Input: part model. Units: mm. Frame: model coordinates. A direction names the side the tool comes from. Coordinates: 2 decimals unless noted, no trailing zeros. Loops run counter-clockwise (first coordinate to the right, second up) from the corner with the lowest first, then second, coordinate; pieces in that order, holes last.
Item 1: Reachability of faces 4 (the flat face through (1, 0, 8)), 5 (the flat face through (0, 3, -5.25)) from +Z, -Z, +X, -X, +Y, -Y: full face, straight path, thin tool, end or side. Return the list, or none.
Item 2: Section B-B on x = 29.75. Return loops of the section in (y, z), and give its area (3 significant figures).
Item 3: Section D-D on x = -16.5. Return loops of the section in (y, z).
Item 4: Section C-C on y = 2.2. Return loops of the section in (x, z), and give its area (3 significant figures).
Item 5: Section A-A on z = 0. Return loops of the section in (x, y), and give its area (3 significant figures).
Item 6: Contact query for flat-ended pins moving along their axis: P1, Ø1, axis at x = -44, y = 3.5, coming from the -Z side; P2, Ø1.6, axis at y = 2, z = 2, coming from the -X side; P3, Ø1.5, axis at x = 30, y = 4.5, coming from the -Z side. Output: stop coordinate, or through.
Item 7: Ray query, line 1 along X through (y, z) = (2.4, 0); line 2 along Z through (x, y) = (-3, 0.9); line 3 along Z through (x, y) = (-29.75, 1). Return the intervals inside material, ascending.
Item 8: Pull-direction query (X, two-part tool) for faces 1 (the cylindrical face through (55.322, 4.145, -0.487)), 2 (the flat face through (1, 5.5, 7)), 3 (the cylindrical face through (-27.554, 1.972, -0.488)); classes: released by +X, released by -X, zero draft, split by the parting line, or undercut.
Autodesk Inventor part; units mm, degrees
ref_plane "YZ Plane" through (0, 0, 0) normal (1, 0, 0) x (0, 1, 0)
ref_plane "XZ Plane" through (0, 0, 0) normal (0, 1, 0) x (-1, 0, 0)
ref_plane "XY Plane" through (0, 0, 0) normal (0, 0, 1) x (1, 0, 0)
sketch "Sketch1" plane through (0, 0, 0) normal (0, 1, 0) x (-1, 0, 0)
  line L0 (-56.75, -34.75) -> (56.75, -34.75)
  line L1 (56.75, -34.75) -> (56.75, 34.75)
  line L2 (56.75, 34.75) -> (-56.75, 34.75)
  line L3 (-56.75, 34.75) -> (-56.75, -34.75)
  line L4 (-56.75, -34.75) -> (56.75, 34.75) construction
  line L5 (56.75, -34.75) -> (-56.75, 34.75) construction
  point P0 (0, 0)
  dimension "d0" = 113.5
  dimension "d1" = 69.5
extrude "Extrusion1" add sketch "Sketch1" along normal blind 5.5
sketch "Sketch2" plane through (0, 5.5, 0) normal (0, 1, 0) x (1, 0, 0)
  line L0 (56.75, 34.75) -> (-56.75, 34.75)
  line L1 (-56.75, 34.75) -> (-56.75, -34.75)
  line L2 (-56.75, -34.75) -> (56.75, -34.75)
  line L3 (56.75, -34.75) -> (56.75, 34.75)
  line L4 (11.75, -5.25) -> (-11.75, -5.25)
  line L5 (-11.75, -5.25) -> (-11.75, 5.25)
  line L6 (-11.75, 5.25) -> (11.75, 5.25)
  line L7 (11.75, 5.25) -> (11.75, -5.25)
  line L8 (11.75, -5.25) -> (-11.75, 5.25) construction
  line L9 (-11.75, -5.25) -> (11.75, 5.25) construction
  point P0 (0, 0)
  dimension "d4" = 45
  dimension "d5" = 29.5
extrude "Extrusion2" cut sketch "Sketch2" against normal up to next contours L4 L5 L6 L7
sketch "Sketch3" plane through (0, 5.5, 0) normal (0, 1, 0) x (1, 0, 0)
  line L0 (11.75, 5.25) -> (11.75, -5.25)
  line L1 (11.75, 0) -> (29.75, 0)
  line L2 (-11.75, 5.25) -> (-11.75, -5.25)
  line L3 (-11.75, 0) -> (-29.75, 0)
  point P0 (0, 0)
  dimension "d8" = 18
hole "Hole1" at (-29.75, 5.5, 0) at (29.75, 5.5, 0) direction (0, -1, 0) diameter 4.5 depth 10 tip angle 118 countersink diameter 7.5 countersink angle 90
fillet "Fillet1" radius 4.75 4 edges at (-56.75, 5.5, 0) (56.75, 5.5, 0) (0, 5.5, 34.75) (0, 5.5, -34.75)
properties part number "Plate"
Results found:
1. face 4: +Z, -Z, +X, -X, -Y
1. face 5: +Y, -Y
2. outline: (0, -34.75) - (0.75, -34.75) arc R4.75 ccw to (5.5, -30) - (5.5, -3.75) - (4, -2.25) - (0, -2.25) - close; (0, 2.25) - (4, 2.25) - (5.5, 3.75) - (5.5, 30) arc R4.75 ccw to (0.75, 34.75) - (0, 34.75) - close
2. area: 346 mm2
3. outline: (0, -34.75) - (0.75, -34.75) arc R4.75 ccw to (5.5, -30) - (5.5, 30) arc R4.75 ccw to (0.75, 34.75) - (0, 34.75) - close
4. outline: (-56.52, -34.52) - (56.52, -34.52) - (56.52, 34.52) - (-56.52, 34.52) - close; hole circle Ø4.5 at (-29.75, 0); hole (-11.75, -5.25) - (11.75, -5.25) - (11.75, 5.25) - (-11.75, 5.25) - close; hole circle Ø4.5 at (29.75, 0)
4. area: 7,530 mm2
5. outline: (-56.75, 0) - (-32, 0) - (-32, 4) - (-33.5, 5.5) - (-52, 5.5) arc R4.75 ccw to (-56.75, 0.75) - close; (-27.5, 0) - (-11.75, 0) - (-11.75, 5.5) - (-26, 5.5) - (-27.5, 4) - close; (11.75, 0) - (27.5, 0) - (27.5, 4) - (26, 5.5) - (11.75, 5.5) - close; (32, 0) - (56.75, 0) - (56.75, 0.75) arc R4.75 ccw to (52, 5.5) - (33.5, 5.5) - (32, 4) - close
5. area: 431 mm2
6. P1: stops at z = -34.18
6. P2: stops at x = -56.73
6. P3: stops at z = -33.68
7. line 1: x = -56.45 to -32, -27.5 to -11.75, 11.75 to 27.5, 32 to 56.45
7. line 2: z = -34.75 to -5.25, 5.25 to 34.75
7. line 3: z = -34.74 to -2.25, 2.25 to 34.74
8. face 1: released by +X
8. face 2: zero draft
8. face 3: undercut
